from build123d import *

# Parameters (mm, degrees)
FILLET1_R = 0.5


with BuildPart() as part:
    # Sketch1 → Revolve1 (revolve)
    with BuildSketch(Plane.XY):
        with BuildLine():
            Line((-3.5, 9.5), (-1.677050983, 9.5))
            ThreePointArc((-1.677050983, 9.5), (0, 10.25), (1.677050983, 9.5))
            Line((1.677050983, 9.5), (3.5, 9.5))
            Line((3.5, 9.5), (3.5, 11))
            Line((3.5, 11), (-3.5, 11))
            Line((-3.5, 11), (-3.5, 9.5))
        make_face()
    revolve(axis=Axis((-29.842592593, 0, 0), (1, 0, 0)))

    # Fillet1
    fillet1_edges = [part.edges().sort_by_distance(p)[0] for p in [
        (3.5, -11, 0),
        (-3.5, -11, 0),
    ]]
    fillet(fillet1_edges, radius=FILLET1_R)


solid = part.part
The listing builds one solid part. Answer for the finished solid, in the listing's coordinates (mm). Coordinates: 2 decimals unless noted, no trailing zeros. Loops run counter-clockwise (first coordinate to the right, second up) from the corner with the lowest first, then second, coordinate; pieces in that order, holes last. Notation, with made-up numbers: M 25,50.25 L 34,50.25 A22 cw 34,68.25 Z; hole C 4,8 d11. An arc over 180 degrees is marked long. Answer in a Markdown table with one row per item.
1) Find section C-C (x = 1). Determine the outline of the cut face in (y, z).
Answers below:
| item | result |
|---|---|
| outline | C 0,0 d22; hole C 0,0 d20.03 |
2) Given pin 1 (1 mm diameter, centred on x = -1, y = -2.5, fed in from -Z); pin 2 (5 mm diameter, centred on y = -8.5, z = -1.5, fed in from -X); pin 3 (1.5 mm diameter, centred on x = 0.5, y = -2, fed in from +Z); pin 4 (4 mm diameter, centred on x = 0, y = 5.5, fed in from +Z), each flat-ended and moving along its own axis, determine where each tip first touches the part or whether it passes through.
Answers below:
| item | result |
|---|---|
| pin 1 | z = -10.82 |
| pin 2 | x = -3.5 |
| pin 3 | z = 10.93 |
| pin 4 | z = 10.43 |
3) Find section A-A (z = 0). Determine the outline of the cut face in (x, y), then the cut area to 3 significant figures.
Answers below:
| item | result |
|---|---|
| outline | M -3.5,-10.5 A0.5 ccw -3,-11 L 3,-11 A0.5 ccw 3.5,-10.5 L 3.5,-9.5 L 1.68,-9.5 A2.25 cw -1.68,-9.5 L -3.5,-9.5 Z; M -3.5,9.5 L -1.68,9.5 A2.25 cw 1.68,9.5 L 3.5,9.5 L 3.5,10.5 A0.5 ccw 3,11 L -3,11 A0.5 ccw -3.5,10.5 Z |
| area | 17.3 mm^2 |
4) Find the intervals of material crossed by probe 1 along Z at (x, y) = (2.2, 0); probe 2 along Z at (x, y) = (0.5, -8.75); probe 3 along Y at (x, z) = (-1.25, -7.5), in increasing order.
Answers below:
| item | result |
|---|---|
| probe 1 | -11 to -9.5, 9.5 to 11 |
| probe 2 | -6.67 to -5.23, 5.23 to 6.67 |
| probe 3 | -8.05 to -6.42, 6.42 to 8.05 |
